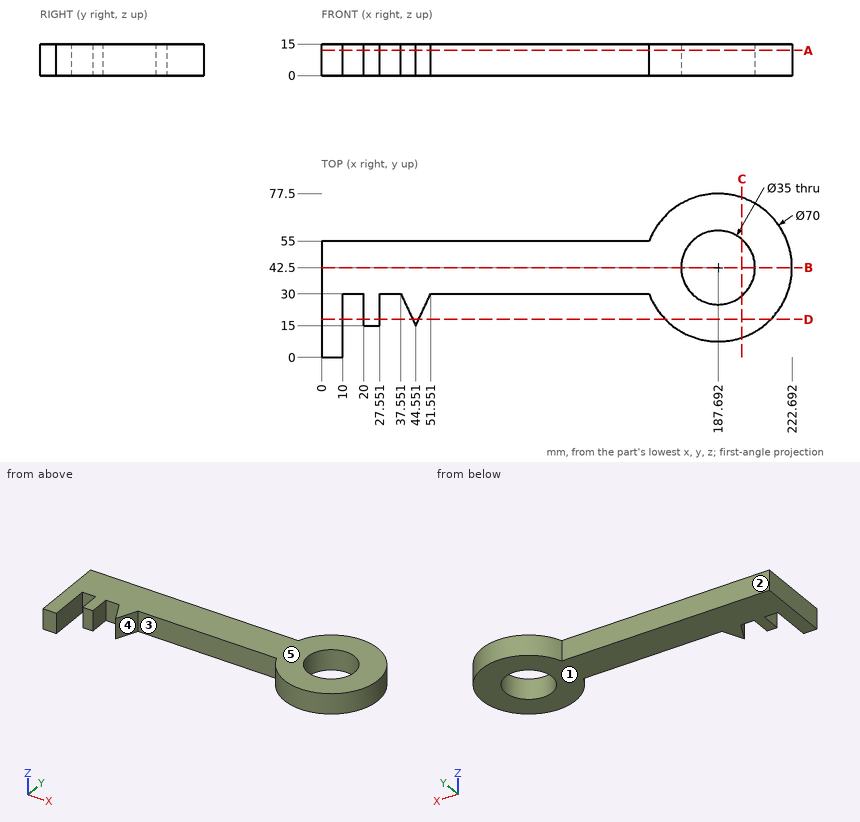
Source: three-view drawing plus pictorial views. Frame: mm from the lowest corner of the part. A direction names the side the tool comes from. Coordinates: 2 decimals unless noted, no trailing zeros. Order: outer loops, then holes, each group sorted by start corner. A loop starts at its lowest first (then second) coordinate and runs counter-clockwise, first axis right, second up. Notation, with made-up numbers: M -36.5,-1 L -1.5,-1 A27 cw -1.5,16 Z; hole C -31.5,5.25 d4. An arc over 180 degrees is marked long. One line per question, with ' | ' between items. Start each with the question number.
Item 1: Cut plane A-A, the plane z = 12. Return the cut outline in (x, y), then the cut area to 3 significant figures.
Item 2: Pin query (flat end, axial travel): pin 1 Ø6 at (x, z) = (41.5, 7.5) entering from +Y; pin 2 Ø3 at (x, z) = (31, 8.5) entering from -Y; pin 3 Ø21 at (x, y) = (187.69, 42.5) entering from -Z; pin 4 Ø8.5 at (x, z) = (25.5, 8.5) entering from -Y. Return the tip coordinate at first contact, or that it passes through.
Item 3: Cut plane C-C, the plane x = 199. Return the cut outline in (y, z) (1 decimal).
Item 4: Set-up query: the marked faces 1, 2 and 3. Return all of +Z, -Z, +X, -X, +Y, -Y with unobstructed straight access to the full face (end or side cutting, diameter ignored); none if empty.
Item 5: Cut plane D-D, the plane y = 18. Return the cut outline in (x, z).
Item 6: Cut plane B-B, the plane y = 42.5. Return the cut outline in (x, z).
Item 7: Draft query along X for the marked faces 4 and 5. Return one class per face: released by +X, released by -X, zero draft, split by the parting line, or undercut.
Item 8: Ray query, probe 1 along X at (y, z) = (43.5, 1.25); probe 2 along Y at (x, z) = (193.5, 10.75) (1 decimal); probe 3 along X at (y, z) = (51, 10) (1 decimal). Return the intervals inside material, ascending. Write a range as [from, to].
A:
1) outline: M 0,0 L 10,0 L 10,30 L 20,30 L 20,15 L 27.55,15 L 27.55,30 L 37.55,30 L 44.55,15 L 51.55,30 L 155,30 A35 ccw long 155,55 L 0,55 Z; hole C 187.69,42.5 d35 | area: 7,240 mm2
2) pin 1: stops at y = 55 | pin 2: stops at y = 30 | pin 3: passes through | pin 4: stops at y = 15
3) outline: M 9.4,0 L 29.1,0 L 29.1,15 L 9.4,15 Z; M 55.9,0 L 75.6,0 L 75.6,15 L 55.9,15 Z
4) face 1: -Z, +X, -X, +Y, -Y | face 2: +Z, -Z, -X, +Y | face 3: +Z, -Z, -Y
5) outline: M 0,0 L 10,0 L 10,15 L 0,15 Z; M 20,0 L 27.55,0 L 27.55,15 L 20,15 Z; M 43.15,0 L 45.95,0 L 45.95,15 L 43.15,15 Z; M 162.7,0 L 212.69,0 L 212.69,15 L 162.7,15 Z
6) outline: M 0,0 L 170.19,0 L 170.19,15 L 0,15 Z; M 205.19,0 L 222.69,0 L 222.69,15 L 205.19,15 Z
7) face 4: undercut | face 5: zero draft
8) probe 1: x = [0, 170.22], [205.16, 222.68] | probe 2: y = [8, 26], [59, 77] | probe 3: x = [0, 172.4], [203, 221.6]
